from build123d import *

# Parameters (mm, degrees)
F0_W      = 92.61
F0_H      = 70.8
F1_DEPTH  = 2
F2_W      = 28
F2_H      = 64.8
F3_DEPTH  = 16
F4_W      = 9.2
F4_H      = 64.8
F5_DEPTH  = 5
F7_W      = 12.25
F7_H      = 15
F8_DEPTH  = 10.75
F9_R      = 1.5
F10_W     = 12.25
F10_H     = 10.75
F11_DEPTH = 2
F12_W     = 10.5
F12_H     = 9
F13_DEPTH = 11.5


# Not quite as in the source:
# - a pattern or mirror of a feature is missing from the dataset's text; its kind, count and spacing are read off the source's solid


with BuildPart() as f1:
    # F0 (on Top) → F1 (new body)
    with BuildSketch(Plane.XY):
        with Locations((46.305, 35.4)):
            Rectangle(F0_W, F0_H)
    extrude(amount=F1_DEPTH)

    # F2 (on face) → F3 (join)
    with BuildSketch(Plane.XY.offset(2)):
        with Locations((78.61, 35.4)):
            Rectangle(F2_W, F2_H)
    f3 = extrude(amount=F3_DEPTH)

    # F3_copies: F3 across plane
    add(f3.mirror(Plane(origin=(46.305, 0, 0), x_dir=(0, 0, -1), z_dir=(-1, 0, 0))))

    # F4 (on face) → F5 (cut)
    with BuildSketch(Plane.XY.offset(18)):
        with Locations((88.01, 35.4)):
            Rectangle(F4_W, F4_H)
    f5 = extrude(amount=-F5_DEPTH, mode=Mode.SUBTRACT)

    # F5_copies: F5 across plane
    add(f5.mirror(Plane(origin=(46.305, 0, 0), x_dir=(0, 0, -1), z_dir=(-1, 0, 0))), mode=Mode.SUBTRACT)

    # F7 (on face) → F8 (join)
    with BuildSketch(Plane.XY.offset(2)):
        with Locations((46.305, 7.5)):
            Rectangle(F7_W, F7_H)
    extrude(amount=F8_DEPTH)

    # F9
    f9_edges = [f1.edges().sort_by_distance(p)[0] for p in [
        (92.61, 70.8, 1),
        (0, 70.8, 1),
        (0, 0, 1),
        (92.61, 0, 1),
    ]]
    fillet(f9_edges, radius=F9_R)

    # F10 (on face) → F11 (join)
    with BuildSketch(Plane.XZ):
        with Locations((46.305, 7.375)):
            Rectangle(F10_W, F10_H)
    extrude(amount=F11_DEPTH)

    # F12 (on face) → F13 (join)
    with BuildSketch(Plane.XY.offset(2)):
        with Locations((46.305, 65.3)):
            Rectangle(F12_W, F12_H)
    extrude(amount=F13_DEPTH)


solid = f1.part
Geometry: final body of the model. Coordinates: model frame, mm. A direction names the side the tool comes from. Round coordinates to 2 decimals unless told otherwise and drop trailing zeros. Loops run counter-clockwise (first coordinate to the right, second up) from the corner with the lowest first, then second, coordinate; pieces in that order, holes last. Notation, with made-up numbers: M 47.5,56.25 L 56.5,56.25 A19 cw 56.5,83.25 Z; hole C 32.25,-25 d4. An arc over 180 degrees is marked long. One line per question, with ' | ' between items.
(1) Material intervals for line 1 along X through (y, z) = (66.5, 3) (3 decimals); line 2 along Y through (x, z) = (41.5, 3); line 3 along X through (y, z) = (40, 15.75), sorted ascending. Write a range as from..to.
Check result:
line 1: x = 0..28, 41.055..51.555, 64.61..92.61 | line 2: y = -2..15, 60.8..69.8 | line 3: x = 9.2..28, 64.61..83.41
(2) Cut plane B-B on z = 15.5. Return the cut outline in (x, y), plus the area to 3 significant figures.
Check result:
outline: M 9.2,3 L 28,3 L 28,67.8 L 9.2,67.8 Z; M 64.61,3 L 83.41,3 L 83.41,67.8 L 64.61,67.8 Z | area: 2,440 mm2
(3) Access query for faces 1 (the flat face through (78, 3, 10)), 2 (the flat face through (46, 69.8, 8)), 3 (the flat face through (14, 67.8, 10)), 4 (the flat face through (78, 67.8, 10)), 5 (the flat face through (5, 36, 13)). Directions: +Z, -Z, +X, -X, +Y, -Y. A direction counts if a zero-diameter tool reaches every point of the face in a straight line with its end or side. Return the directions, or none.
Check result:
face 1: +Z, +X, -Y | face 2: +Z, +X, -X, +Y | face 3: +Z, -X, +Y | face 4: +Z, +X, +Y | face 5: +Z, -X, +Y, -Y
(4) Pull-direction query (X, two-part tool) for faces 6 (the flat face through (40.18, 7, 7)), 7 (the flat face through (9.2, 35, 16)), 8 (the flat face through (88, 36, 13)), 9 (the flat face through (64.61, 35, 10)); classes: +X half, -X half, draft (parallel to the pull), parting line (faces both ways), or undercut.
Check result:
face 6: undercut | face 7: -X half | face 8: draft | face 9: undercut
(5) Cut plane D-D on y = 44. Return the cut outline in (x, z).
Check result:
outline: M 0,0 L 92.61,0 L 92.61,13 L 83.41,13 L 83.41,18 L 64.61,18 L 64.61,2 L 28,2 L 28,18 L 9.2,18 L 9.2,13 L 0,13 Z
(6) Cut plane C-C on z = 5.25. Return the cut outline in (x, y) (3 decimals), plus the area to 3 significant figures.
Check result:
outline: M 0,3 L 28,3 L 28,67.8 L 0,67.8 Z; M 40.18,-2 L 52.43,-2 L 52.43,15 L 40.18,15 Z; M 41.055,60.8 L 51.555,60.8 L 51.555,69.8 L 41.055,69.8 Z; M 64.61,3 L 92.61,3 L 92.61,67.8 L 64.61,67.8 Z | area: 3,930 mm2
(7) Contact query for flat-ended pins moving along their axis: P1, Ø2.5, axis at y = 41.5, z = 16, coming from the -X side; P2, Ø1.6, axis at x = 63.5, z = 1, coming from the -Y side; P3, Ø6, axis at x = 48.5, y = 10.5, coming from the +Z side; P4, Ø1, axis at y = 60.5, z = 2.5, coming from the -X side. Output: stop coordinate, or through.
Check result:
P1: stops at x = 9.2 | P2: stops at y = 0 | P3: stops at z = 12.75 | P4: stops at x = 0
(8) Cut plane A-A on x = 46. Return the cut outline in (y, z), plus the area to 3 significant figures.
Check result:
outline: M -2,2 L 0,2 L 0,0 L 70.8,0 L 70.8,2 L 69.8,2 L 69.8,13.5 L 60.8,13.5 L 60.8,2 L 15,2 L 15,12.75 L -2,12.75 Z | area: 428 mm2
